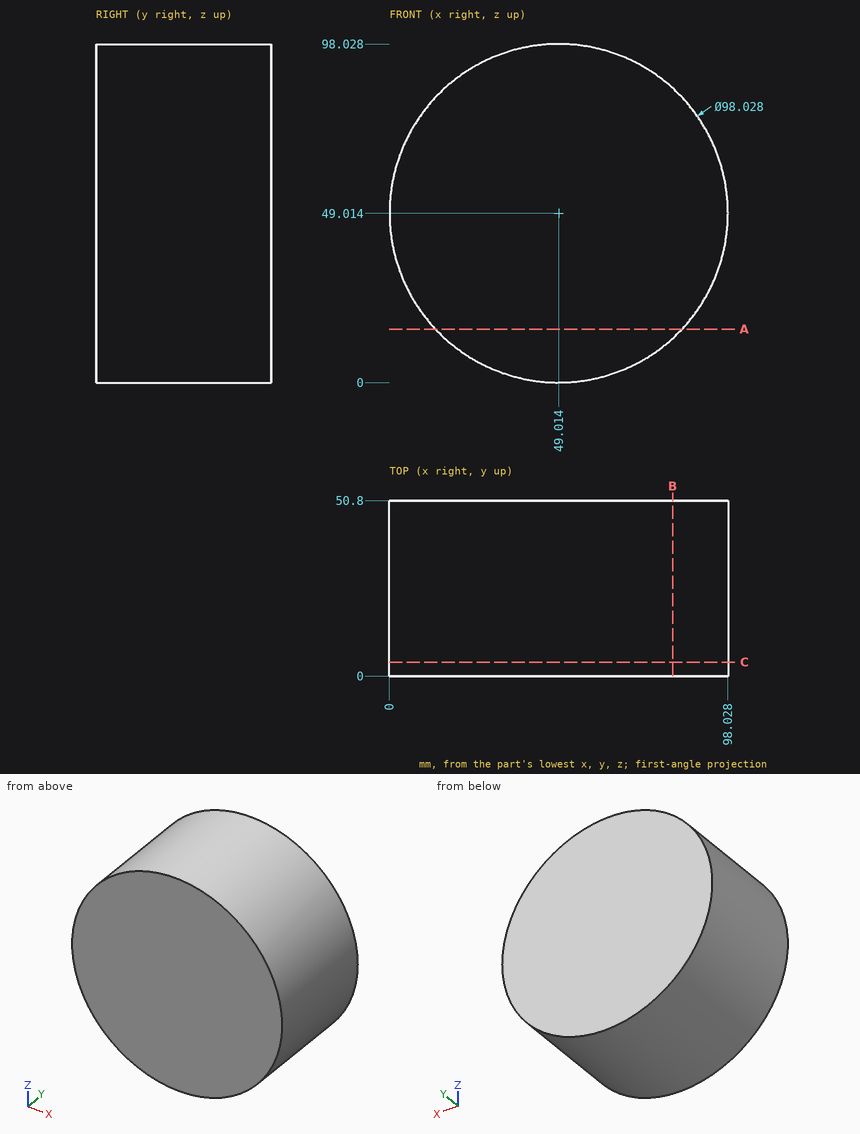
Input: dimensioned drawing with shaded views. Units: mm. Origin: part minimum x, y, z. Give positions to 0.01 mm unless a question says otherwise; leave off trailing zeros. Write each loop counter-clockwise with the first axis right and the second up, starting at its lowest first coordinate (ties: lowest second). Pieces come first, ordered by that corner, then holes. Notation, with made-up numbers: (25.25, 30) -> (70.25, 30) arc R17 ccw to (70.25, 44) -> close; hole circle Ø11 at (-13, -8.75). An arc over 180 degrees is marked (long way). Answer as a JSON object with one key per item and string values.
1. Contact query for flat-ended pins moving along their axis: pin 1 (6 mm diameter, centred on x = 26.5, y = 36, fed in from -Z); pin 2 (6 mm diameter, centred on y = 30, z = 81, fed in from -X); pin 3 (12 mm diameter, centred on x = 52.5, y = 19.5, fed in from -Z). Output: stop coordinate, or through.
Ans:
{"pin 1": "stops at z = 4.05", "pin 2": "stops at x = 9.49", "pin 3": "stops at z = 0"}
2. Cut plane A-A on z = 15.5. Output: boundary loops of the cut face in (x, y), and give its area (3 significant figures).
Ans:
{"outline": "(13.25, 0) -> (84.78, 0) -> (84.78, 50.8) -> (13.25, 50.8) -> close", "area": "3,630 mm^2"}
3. Cut plane B-B on x = 82. Output: boundary loops of the cut face in (y, z), and give its area (3 significant figures).
Ans:
{"outline": "(0, 12.76) -> (50.8, 12.76) -> (50.8, 85.27) -> (0, 85.27) -> close", "area": "3,680 mm^2"}
4. Ray query, probe 1 along Z at (x, y) = (48.5, 7); probe 2 along X at (y, z) = (23, 28.5); probe 3 along Z at (x, y) = (66, 44). Return the intervals inside material, ascending. Write a range as from..to.
Ans:
{"probe 1": "z = 0..98.03", "probe 2": "x = 4.5..93.53", "probe 3": "z = 3.04..94.99"}
5. Cut plane C-C on y = 4. Output: boundary loops of the cut face in (x, z), and give its area (3 significant figures).
Ans:
{"outline": "circle Ø98.03 at (49.01, 49.01)", "area": "7,550 mm^2"}
